from build123d import *

# Parameters (mm, degrees)
BOSS_EXTRUDE1_DEPTH = 18
SKETCH3_R           = 1.6
CUT_EXTRUDE1_DEPTH  = 56.244999774
SKETCH5_W           = 22.958144304
SKETCH5_H           = 5
BOSS_EXTRUDE2_DEPTH = 5
SKETCH6_R           = 8.025
CUT_EXTRUDE2_DEPTH  = 57.329388422
SKETCH7_R           = 9
SKETCH7_R_2         = 7
BOSS_EXTRUDE3_DEPTH = 1
FILLET1_R           = 7
FILLET2_R           = 10
BOSS_EXTRUDE4_DEPTH = 12
SKETCH9_R           = 1.45
CUT_EXTRUDE3_DEPTH  = 4.15


with BuildPart() as part:
    # Sketch1 → Boss-Extrude1 (new body)
    with BuildSketch(Plane.XY):
        with BuildLine():
            Line((15.267285286, 1), (28.676455767, 1))
            Line((28.676455767, 1), (28.676455767, 4))
            Line((28.676455767, 4), (18.676455767, 4))
            ThreePointArc((18.676455767, 4), (5.072789326, 18.414038353), (-13.99321264, 13))
            Line((-13.99321264, 13), (-50, 13))
            Line((-50, 13), (-50, 8))
            Line((-50, 8), (-13.041855696, 8))
            ThreePointArc((-13.041855696, 8), (3.67261953, 14.852672008), (15.267285286, 1))
        make_face()
    extrude(amount=BOSS_EXTRUDE1_DEPTH)

    # Sketch3 → Cut-Extrude1 (cut, through all)
    with BuildSketch(Plane(origin=(0, 4, 0), x_dir=(1, 0, 0), z_dir=(0, 1, 0))):
        with Locations(Location((23.676455767, -4, 0), (0, 0, 270))):
            Circle(SKETCH3_R)
        with Locations(Location((23.676455767, -14, 0), (0, 0, 270))):
            Circle(SKETCH3_R)
    extrude(amount=-CUT_EXTRUDE1_DEPTH, mode=Mode.SUBTRACT)

    # Sketch5 → Boss-Extrude2 (add)
    with BuildSketch(Plane.XZ.offset(-8)):
        with Locations((-38.520927848, 20.5)):
            Rectangle(SKETCH5_W, SKETCH5_H)
    extrude(amount=-BOSS_EXTRUDE2_DEPTH)

    # Sketch6 → Cut-Extrude2 (cut, through all)
    with BuildSketch(Plane(origin=(0, 13, 0), x_dir=(1, 0, 0), z_dir=(0, 1, 0))):
        with Locations(Location((-37, -12, 0), (0, 0, 180))):
            Circle(SKETCH6_R)
    extrude(amount=-CUT_EXTRUDE2_DEPTH, mode=Mode.SUBTRACT)

    # Sketch7 → Boss-Extrude3 (add)
    with BuildSketch(Plane.XZ.offset(-8)):
        with Locations(Location((-37, 12, 0), (0, 0, 180))):
            Circle(SKETCH7_R)
        with Locations((-37, 12)):
            Circle(SKETCH7_R_2, mode=Mode.SUBTRACT)
    extrude(amount=BOSS_EXTRUDE3_DEPTH)

    # Fillet1
    fillet1_edges = [part.edges().sort_by_distance(p)[0] for p in [
        (-50, 10.5, 23),
        (-50, 10.5, 0),
    ]]
    fillet(fillet1_edges, radius=FILLET1_R)

    # Fillet2
    # the kernel refuses this fillet: 10 mm, written as the material it takes off along each edge
    with BuildSketch(Plane(origin=(-27.041855696, -13.650635095, 23), x_dir=(0, 0, -1), z_dir=(0, 1, 0))) as fillet2_piece_1:
        with BuildLine():
            CenterArc((10, 8.660254038), FILLET2_R, 180, 60)
            Line((0, 8.660254038), (-0.2, 8.660254038))
            Line((-0.2, 8.660254038), (-0.2, 0))
            Line((-0.2, 0), (0, -0.2))
            ThreePointArc((0, -0.2), (2.5, -0.2), (4.9, -0.173205081))
            Line((4.9, -0.173205081), (5, 0))
        make_face()
    extrude(amount=48.301270189, mode=Mode.SUBTRACT)

    # Sketch8 → Boss-Extrude4 (add)
    with BuildSketch(Plane.XY.offset(18)):
        Polygon((6, 18.133118871), (6, 19.3), (-5.66, 19.3), (-5.66, 18.242105142), align=None)
    extrude(amount=-BOSS_EXTRUDE4_DEPTH)

    # Sketch9 → Cut-Extrude3 (cut)
    with BuildSketch(Plane(origin=(0, 19.3, 0), x_dir=(1, 0, 0), z_dir=(0, 1, 0))):
        with Locations(Location((0, -15, 0), (0, 0, 270))):
            Circle(SKETCH9_R)
        with Locations(Location((0, -9, 0), (0, 0, 270))):
            Circle(SKETCH9_R)
    extrude(amount=-CUT_EXTRUDE3_DEPTH, mode=Mode.SUBTRACT)


solid = part.part
Source: CAD feature listing. Evaluate the final solid. Frame: model axes, mm. A direction names the side the tool comes from. Give positions to 0.01 mm unless a question says otherwise; leave off trailing zeros. Write each loop counter-clockwise with the first axis right and the second up, starting at its lowest first coordinate (ties: lowest second). Pieces come first, ordered by that corner, then holes. Notation, with made-up numbers: M 81.5,34 L 110.5,34 A19 ccw 110.5,66 Z; hole C 1.25,78.5 d10. An arc over 180 degrees is marked long. Return JSON: item names as keys, results as strings. Group by question number.
1) Cut plane C-C, the plane x = 24.5. Output: boundary loops of the cut face in (y, z).
2) Ray query, L1, parallel to Z at x = 0, y = 17; L2, parallel to X at y = 7.5, z = 16; L3, parallel to Z at x = -37, y = 9.5 (3 decimals). Return the intervals inside material, ascending.
3) Cut plane A-A, the plane x = -37. Output: boundary loops of the cut face in (y, z) (3 decimals), then the cut area to 4 significant figures.
4) Cut plane B-B, the plane y = 8.75. Output: boundary loops of the cut face in (x, z) (3 decimals), then the cut area to 3 significant figures.
5) First-contact query: pin 1 Ø5 at (x, z) = (-39.5, 16) entering from +Y; pin 2 Ø10 at (x, z) = (17, 6.5) entering from +Y; pin 3 Ø2 at (x, z) = (-23, 6.5) entering from +Y. Flat tips, straight axial feed; report the tip coordinate or a pass-through.
6) Cut plane D-D, the plane x = -16.5. Output: boundary loops of the cut face in (y, z), then the cut area to 3 significant figures.
7) Draft query along Z for faces 1 (the face through (1, 16, 18)), 2 (the face through (-29.86, 7.51, 17.48)), 3 (the face through (-35, 8, 5)), 4 (the face through (0, 19.3, 12)). Return one class per face: released by +Z, released by -Z, zero draft, split by the parting line, or undercut.
8) Set-up query: faces 5 (the face through (-44.654, 10.535, 14.41)), 6 (the face through (24, 4, 9)), 7 (the face through (-28, 13, 9)), 8 (the face through (28.676, 2, 9)). Return all of +Z, -Z, +X, -X, +Y, -Y with unobstructed straight access to the full face (end or side cutting, diameter ignored); none if empty.
Data:
{
 "1": {"outline": "M 1,0 L 4,0 L 4,2.63 L 1,2.63 Z; M 1,5.37 L 4,5.37 L 4,12.63 L 1,12.63 Z; M 1,15.37 L 4,15.37 L 4,18 L 1,18 Z"},
 "2": {"L1": "z = 0 to 7.55, 10.45 to 13.55, 16.45 to 18", "L2": "x = -45.06 to -42.74, -31.26 to -28.94, 13.34 to 17.57", "L3": "z = 0 to 3.975, 20.025 to 23"},
 "3": {"outline": "M 7,3 L 8,3 L 8,0 L 13,0 L 13,3.975 L 8,3.975 L 8,5 L 7,5 Z; M 7,19 L 8,19 L 8,20.025 L 13,20.025 L 13,23 L 8,23 L 8,21 L 7,21 Z", "area": "38.75 mm²"},
 "4": {"outline": "M -50,7 A7 ccw -43,0 L -12.551,0 L -12.551,18 L -27.042,18 A10 ccw -35.702,23 L -43,23 A7 ccw -50,16 Z; M 12.551,0 L 16.978,0 L 16.978,18 L 12.551,18 Z; hole C -37,12 d16.05", "area": "633 mm²"},
 "5": {"pin 1": "stops at y = 8", "pin 2": "stops at y = 14.86", "pin 3": "stops at y = 13"},
 "6": {"outline": "M 8,0 L 13,0 L 13,18 L 8,18 Z", "area": "90.0 mm²"},
 "7": {"face 1": "released by +Z", "face 2": "split by the parting line", "face 3": "undercut", "face 4": "zero draft"},
 "8": {"face 5": "+Y", "face 6": "+Z, -Z, +X, +Y", "face 7": "+Z, -Z, -X, +Y", "face 8": "+Z, -Z, +X, +Y, -Y"}
}
